CAD build for the part. Positions are in the model's coordinates, mm. A direction names the side the tool comes from. Round coordinates to 2 decimals unless told otherwise and drop trailing zeros. Order: outer loops, then holes, each group sorted by start corner. A loop starts at its lowest first (then second) coordinate and runs counter-clockwise, first axis right, second up.
```python
from build123d import *

# Parameters (mm, degrees)
F0_R     = 1.4351
F1_DEPTH = 2.286
F2_W     = 5.08
F2_H     = 10.621818
F3_DEPTH = 1.143


with BuildPart() as f1:
    # F0 (on Top) → F1 (new body)
    with BuildSketch(Plane.XY):
        with BuildLine():
            ThreePointArc((-2.54, 4.252614), (-5.951509, 3.434359), (-9.144, 1.979734))
            ThreePointArc((-9.144, 1.979734), (-10.239018, -0.46591), (-8.259002, -2.271394))
            Line((-8.259002, -2.271394), (-2.54, -2.921))
            Line((-2.54, -2.921), (-2.54, 4.252614))
        make_face()
        with Locations((-8.001, 0)):
            Circle(F0_R, mode=Mode.SUBTRACT)
        with BuildLine():
            ThreePointArc((2.54, 4.252614), (0, 4.429861), (-2.54, 4.252614))
            Line((-2.54, 4.252614), (-2.54, -2.921))
            Line((-2.54, -2.921), (2.54, -2.921))
            Line((2.54, -2.921), (2.54, 4.252614))
        make_face()
        with BuildLine():
            ThreePointArc((9.144, 1.979734), (5.951509, 3.434359), (2.54, 4.252614))
            Line((2.54, 4.252614), (2.54, -2.921))
            Line((2.54, -2.921), (8.259002, -2.271394))
            ThreePointArc((8.259002, -2.271394), (10.239018, -0.46591), (9.144, 1.979734))
        make_face()
        with Locations((8.001, 0)):
            Circle(F0_R, mode=Mode.SUBTRACT)
    extrude(amount=F1_DEPTH)

    # F2 (on face) → F3 (cut)
    with BuildSketch(Plane.XY.offset(2.286)):
        with Locations((0, 0.276294)):
            Rectangle(F2_W, F2_H)
    extrude(amount=-F3_DEPTH, mode=Mode.SUBTRACT)


solid = f1.part
```
1. Cut at A-A, the plane z = 1.7. Write the cut outline in (x, y).
2. Tool access for faces 1 (the face through (-2.54, 1, 2)), 2 (the face through (-5.44, -2.59, 1.13)): list every direction of +Z, -Z, +X, -X, +Y, -Y with a clear straight run to the whole face (end or side of a thin tool).
3. Drill centre lines: line 1 (X direction, y = 0.5, z = 0.2); line 2 (X direction, y = -0.75, z = 2.05); line 3 (X direction, y = -1, z = 1.75). Where is each one in solid material? Low to high.
4. Mould opens along X. For faces 3 (the face through (5.998, 3.418, 1.127)), 4 (the face through (-6.63, 0.43, 1.13)), 5 (the face through (0, 1, 1.143)), 6 (the face through (0, 1, 0)) say: released by +X, released by -X, zero draft, split by the parting line, or undercut.
5. Pin check, flat tips, straight feed: P1, Ø2.5, axis at x = 8.001, y = 0, coming from the +Z side; P2, Ø3, axis at x = 7.5, y = 3, coming from the +Z side; P3, Ø0.9, axis at y = 1.5, z = 1.5, coming from the -X side; P4, Ø0.9, axis at y = -1, z = 2, coming from the +X side. Stop position of each tip, or through.
6. Cut at C-C, the plane x = -6.75. Write the cut outline in (y, z), and give its area (3 significant figures).
7. Cut at D-D, the plane z = 0.5. Write the cut outline in (x, y).
8. Cut at B-B, the plane y = 0. Write the cut outline in (x, z), and give its area (3 significant figures).
Outcome:
1. outline: (-9.14, 1.98) arc R2.29 ccw to (-8.26, -2.27) - (-2.54, -2.92) - (-2.54, 4.25) arc R18.29 ccw to start; (2.54, -2.92) - (8.26, -2.27) arc R2.29 ccw to (9.14, 1.98) arc R18.29 ccw to (2.54, 4.25) - close; hole circle Ø2.87 at (-8, 0); hole circle Ø2.87 at (8, 0)
2. face 1: +Z, +Y, -Y
2. face 2: +Z, -Z, -X, -Y
3. line 1: x = -10.23 to -9.35, -6.66 to 6.66, 9.35 to 10.23
3. line 2: x = -10.16 to -9.22, -6.78 to -2.54, 2.54 to 6.78, 9.22 to 10.16
3. line 3: x = -10.06 to -9.03, -6.97 to -2.54, 2.54 to 6.97, 9.03 to 10.06
4. face 3: released by +X
4. face 4: undercut
4. face 5: undercut
4. face 6: zero draft
5. P1: passes through
5. P2: stops at z = 2.29
5. P3: stops at x = -10.03
5. P4: stops at x = 10.22
6. outline: (-2.44, 0) - (-0.7, 0) - (-0.7, 2.29) - (-2.44, 2.29) - close; (0.7, 0) - (3.14, 0) - (3.14, 2.29) - (0.7, 2.29) - close
6. area: 9.54 mm2
7. outline: (-9.14, 1.98) arc R2.29 ccw to (-8.26, -2.27) - (-2.54, -2.92) - (2.54, -2.92) - (8.26, -2.27) arc R2.29 ccw to (9.14, 1.98) arc R18.29 ccw to (2.54, 4.25) arc R18.29 ccw to (-2.54, 4.25) arc R18.29 ccw to start; hole circle Ø2.87 at (-8, 0); hole circle Ø2.87 at (8, 0)
8. outline: (-10.29, 0) - (-9.44, 0) - (-9.44, 2.29) - (-10.29, 2.29) - close; (-6.57, 0) - (6.57, 0) - (6.57, 2.29) - (2.54, 2.29) - (2.54, 1.14) - (-2.54, 1.14) - (-2.54, 2.29) - (-6.57, 2.29) - close; (9.44, 0) - (10.29, 0) - (10.29, 2.29) - (9.44, 2.29) - close
8. area: 28.1 mm2
